from build123d import *

# Parameters (mm, degrees)
EXTRUDE_1_DEPTH          = 12
SKETCH_3_R               = 1.5
CUT_EXTRUDE_1_DEPTH      = 39
CUT_EXTRUDE_START        = -6
SKETCH_4_R               = 3.5
CUT_EXTRUDE_2_DEPTH      = 33
SKETCH_5_R               = 3.5
CUT_EXTRUDE_4_DEPTH      = 33
CUT_EXTRUDE_6_DEPTH      = 39
CUT_EXTRUDE_6_DEPTH_BACK = 4
CUT_EXTRUDE_7_DEPTH      = 39
CUT_EXTRUDE_7_DEPTH_BACK = 3


with BuildPart() as part:
    # Эскиз2 → Бобышка-Вытянуть1 (new body)
    with BuildSketch(Plane(origin=(0, 0, 0), x_dir=(1, 0, 0), z_dir=(0, 1, 0))):
        with BuildLine():
            Line((0, 0), (0, 8))
            Line((0, 8), (9, 12))
            Line((9, 12), (25, 12))
            Line((25, 12), (34, 8))
            Line((34, 8), (34, 0))
            Line((34, 0), (23, 0))
            ThreePointArc((23, 0), (17, 6), (11, 0))
            Line((11, 0), (0, 0))
        make_face()
    extrude(amount=EXTRUDE_1_DEPTH)

    # Эскиз3 → Вырез-Вытянуть1 (cut, through all)
    with BuildSketch(Plane.XY):
        with Locations((4.5, 6)):
            Circle(SKETCH_3_R)
        with Locations((29.5, 6)):
            Circle(SKETCH_3_R)
    extrude(amount=-CUT_EXTRUDE_1_DEPTH, mode=Mode.SUBTRACT)

    # Эскиз4 → Вырез-Вытянуть2 (cut, through all)
    with BuildSketch(Plane.XY.offset(CUT_EXTRUDE_START)):
        with Locations((4.5, 6)):
            Circle(SKETCH_4_R)
    extrude(amount=-CUT_EXTRUDE_2_DEPTH, mode=Mode.SUBTRACT)

    # Эскиз5 → Вырез-Вытянуть4 (cut, through all)
    with BuildSketch(Plane.XY.offset(CUT_EXTRUDE_START)):
        with Locations((29.5, 6)):
            Circle(SKETCH_5_R)
    extrude(amount=-CUT_EXTRUDE_4_DEPTH, mode=Mode.SUBTRACT)

    # Эскиз6 → Вырез-Вытянуть6 (cut, two sides: drawn at the far end of the back side and taken through both)
    with BuildSketch(Plane(origin=(0, 12, 0), x_dir=(1, 0, 0), z_dir=(0, 1, 0)).offset(-CUT_EXTRUDE_6_DEPTH_BACK)):
        with BuildLine():
            Line((9, -65.461698495), (9, 0))
            ThreePointArc((9, 0), (17, 8), (25, 0))
            Line((25, 0), (25, -65.461698495))
            Line((25, -65.461698495), (25, -196.385095486))
            Line((25, -196.385095486), (9, -196.385095486))
            Line((9, -196.385095486), (9, -65.461698495))
        make_face()
    extrude(amount=CUT_EXTRUDE_6_DEPTH + CUT_EXTRUDE_6_DEPTH_BACK, mode=Mode.SUBTRACT)

    # Эскиз7 → Вырез-Вытянуть7 (cut, two sides: drawn at the far end of the back side and taken through both)
    with BuildSketch(Plane(origin=(0, 0, 0), x_dir=(-1, 0, 0), z_dir=(0, -1, 0)).offset(-CUT_EXTRUDE_7_DEPTH_BACK)):
        with BuildLine():
            Line((-9, -65.461698495), (-9, 0))
            ThreePointArc((-9, 0), (-17, 8), (-25, 0))
            Line((-25, 0), (-25, -65.461698495))
            Line((-25, -65.461698495), (-25, -196.385095486))
            Line((-25, -196.385095486), (-9, -196.385095486))
            Line((-9, -196.385095486), (-9, -65.461698495))
        make_face()
    extrude(amount=CUT_EXTRUDE_7_DEPTH + CUT_EXTRUDE_7_DEPTH_BACK, mode=Mode.SUBTRACT)


solid = part.part
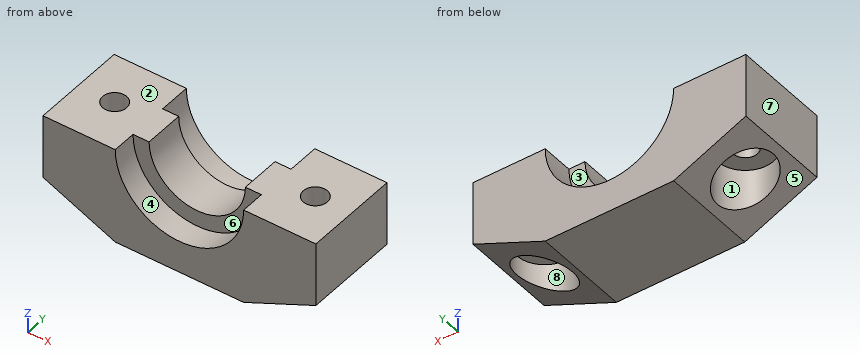
For this review, take the finished solid that the model builds, in its own axes (mm). Face numbers are marked on the shaded views. A direction names the side the tool comes from. Coordinates: 2 decimals unless noted, no trailing zeros. Loops run counter-clockwise (first coordinate to the right, second up) from the corner with the lowest first, then second, coordinate; pieces in that order, holes last. Notation, with made-up numbers: (-7.75, -15) -> (13.25, -15) arc R28 cw to (13.25, 9) -> close; hole circle Ø3 at (-1, 69). An arc over 180 degrees is marked (long way). Write each question's results on one line, items separated by ' | '.
Q1. Mouldability with a two-part tool opening along Y and no side actions: class the marked faces 6, 7 and 8 as +Y half, -Y half, draft (parallel to the pull), parting line (faces both ways), or undercut.
Taken from the geometry:
face 6: -Y half | face 7: draft | face 8: undercut
Q2. Add section A-A, the plane x = 4.5. State the section outline as (y, z) points, then the cut area to 3 significant figures.
Taken from the geometry:
outline: (0, -10) -> (2.5, -10) -> (2.5, -6) -> (4.5, -6) -> (4.5, 0) -> (0, 0) -> close; (7.5, -6) -> (9.5, -6) -> (9.5, -10) -> (12, -10) -> (12, 0) -> (7.5, 0) -> close | area: 74.0 mm²
Q3. Add section B-B, the plane z = -1.75. State the section outline as (x, y) points, then the cut area to 3 significant figures.
Taken from the geometry:
outline: (0, 0) -> (9.19, 0) -> (9.19, 3) -> (11.26, 3) -> (11.26, 8) -> (9.19, 8) -> (9.19, 12) -> (0, 12) -> close; (22.74, 3) -> (24.81, 3) -> (24.81, 0) -> (34, 0) -> (34, 12) -> (24.81, 12) -> (24.81, 8) -> (22.74, 8) -> close; hole circle Ø3 at (4.5, 6); hole circle Ø3 at (29.5, 6) | area: 227 mm²
Q4. For pin 1 Ø3.5 at (x, y) = (30.5, 6) entering from -Z; pin 2 Ø1.5 at (y, z) = (4, -10.5) entering from -X; pin 3 Ø1 at (x, z) = (23.5, -3) entering from +Y, all flat-tipped, find the tip position at first contact; note any pin that passes through.
Taken from the geometry:
pin 1: z = -6 | pin 2: x = 6.67 | pin 3: y = 8
Q5. Add section D-D, the plane z = -6.5. State the section outline as (x, y) points, then the cut area to 3 significant figures.
Taken from the geometry:
outline: (0, 0) -> (12.34, 0) -> (12.34, 3) -> (21.66, 3) -> (21.66, 0) -> (34, 0) -> (34, 12) -> (21.66, 12) -> (21.66, 8) -> (12.34, 8) -> (12.34, 12) -> (0, 12) -> close; hole circle Ø7 at (4.5, 6); hole circle Ø7 at (29.5, 6) | area: 266 mm²
Q6. Machinability: for the marked faces 1, 2, 3, 4 and 5, which of the approach directions +Z, -Z, +X, -X, +Y, -Y give a long, thin tool a straight path to every point of the face, cutting with its end or side? Answer none if there is none.
Taken from the geometry:
face 1: -Z | face 2: +Z, +X, -X, +Y, -Y | face 3: +Z, +Y | face 4: +Z, -Y | face 5: -Z, -X, +Y, -Y
Q7. To check wall thickness, follow line 1 along X through (y, z) = (3.75, -8.5) (3 decimals); line 2 along Y through (x, z) = (4.5, -3.55); line 3 along X through (y, z) = (5.25, -1.75). State the ranges of each line that lie inside material, in increasing order. Write a range as [from, to].
Taken from the geometry:
line 1: [1.125, 1.819], [7.181, 26.819], [32.181, 32.875] | line 2: [0, 4.5], [7.5, 12] | line 3: [0, 3.2], [5.8, 11.26], [22.74, 28.2], [30.8, 34]
Q8. Add section C-C, the plane y = 5.5. State the section outline as (x, z) points, then the cut area to 3 significant figures.
Taken from the geometry:
outline: (0, -8) -> (1.04, -8.46) -> (1.04, -6) -> (3.09, -6) -> (3.09, 0) -> (0, 0) -> close; (5.91, -6) -> (7.96, -6) -> (7.96, -11.54) -> (9, -12) -> (25, -12) -> (26.04, -11.54) -> (26.04, -6) -> (28.09, -6) -> (28.09, 0) -> (23, 0) arc R6 cw to (11, 0) -> (5.91, 0) -> close; (30.91, -6) -> (32.96, -6) -> (32.96, -8.46) -> (34, -8) -> (34, 0) -> (30.91, 0) -> close | area: 226 mm²
